Source: CAD feature listing. Evaluate the final solid. Frame: model axes, mm. Round coordinates to 2 decimals unless told otherwise and drop trailing zeros. Order: outer loops, then holes, each group sorted by start corner. A loop starts at its lowest first (then second) coordinate and runs counter-clockwise, first axis right, second up. Notation, with made-up numbers: (23, 52) - (58, 52) arc R20 cw to (58, 63) - close; hole circle Ø1 at (85, 87.5). An arc over 180 degrees is marked (long way). Put each result on its own line as item: value. Start each with the question number.
1) Line query: probe 1 along Z at (x, y) = (74.25, -88.5); probe 2 along X at (y, z) = (-58.5, 60); probe 3 along Y at (x, z) = (65.75, 38). Output: solid intervals per line, ascending. Write a range as [from, to].
2) Section A-A on y = -99. Output: boundary loops of the cut face in (x, z), then the cut area to 3 significant figures.
3) Section B-B on z = 41.75. Output: boundary loops of the cut face in (x, y).
4) Section D-D on y = -8. Output: boundary loops of the cut face in (x, z), then the cut area to 3 significant figures.
5) Contact query for flat-ended pins moving along their axis: P1, Ø1.5, axis at x = 69.5, z = 25.5, coming from the +Y side; P2, Ø2, axis at x = 63, y = 5, coming from the -Z side; P3, Ø1.3, axis at x = 65.5, y = -112.5, coming from the +Z side; P4, Ø9, axis at x = 65, z = 42, coming from the +Y side. Output: stop coordinate, or through.
6) Section C-C on z = 79.5. Output: boundary loops of the cut face in (x, y), then the cut area to 3 significant figures.
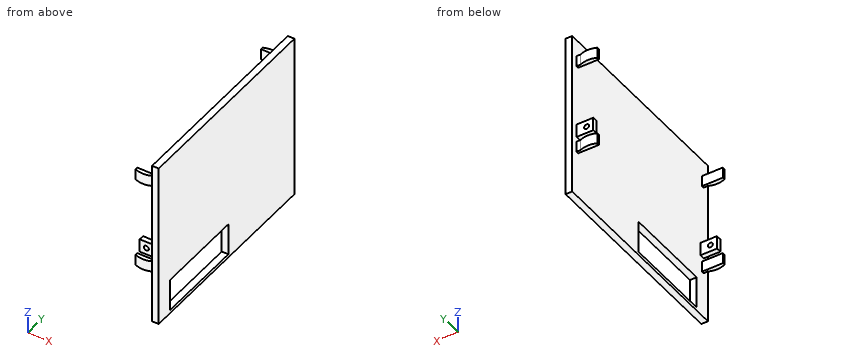
```python
from build123d import *

# Parameters (mm, degrees)
SKETCH2_W               = 4
SKETCH2_H               = 125
BOSS_EXTRUDE2_DEPTH     = 100
CUT_EXTRUDE1_REACH      = 132.347
SKETCH6_W               = 53.8
SKETCH6_H               = 19.347608653
SKETCH9_W               = 6.5
SKETCH9_H               = 1.5
BOSS_EXTRUDE4_DEPTH     = 12.5
BOSS_EXTRUDE5_DEPTH     = 6.5
LPATTERN2_COUNT         = 2
LPATTERN2_PITCH         = 55
MIRROR1_COPY_1_SKETCH_W = 6.5
MIRROR1_COPY_1_SKETCH_H = 1.5
MIRROR1_COPY_1_DEPTH    = 12.5
MIRROR1_COPY_2_DEPTH    = 6.5
SKETCH11_W              = 8
SKETCH11_H              = 3
BOSS_EXTRUDE6_DEPTH     = 10
SKETCH12_R              = 1.5
CUT_EXTRUDE2_DEPTH      = 3


with BuildPart() as part:
    # Sketch2 → Boss-Extrude2 (new body)
    with BuildSketch(Plane.XY):
        with Locations((72.870528802, -53.540266993)):
            Rectangle(SKETCH2_W, SKETCH2_H)
    extrude(amount=BOSS_EXTRUDE2_DEPTH)

    # Sketch6 → Cut-Extrude1 (cut, up to next)
    with BuildSketch(Plane(origin=(70.870528802, -52.340678406, -13.65152284), x_dir=(0, 1, 0), z_dir=(-1, 0, 0)), mode=Mode.PRIVATE) as cut_extrude1_sk1:
        with Locations((-26.429588587, -25.325327166)):
            Rectangle(SKETCH6_W, SKETCH6_H)
    cut_extrude1_tool1 = extrude(cut_extrude1_sk1.sketch, amount=-CUT_EXTRUDE1_REACH, mode=Mode.PRIVATE) & part.part
    add(cut_extrude1_tool1.solids().sort_by_distance((70.870529, -78.770267, 11.673804))[0], mode=Mode.SUBTRACT)

    # Sketch9 → Boss-Extrude4 (add)
    with BuildSketch(Plane.ZY.offset(-70.870528802)):
        with Locations((86.5, -111.290266993)):
            Rectangle(SKETCH9_W, SKETCH9_H)
    boss_extrude4 = extrude(amount=BOSS_EXTRUDE4_DEPTH)

    # Sketch10 → Boss-Extrude5 (add)
    with BuildSketch(Plane.XY.offset(89.75)):
        with BuildLine():
            Line((58.370528802, -112.040266993), (68.370528802, -112.040266993))
            ThreePointArc((68.370528802, -112.040266993), (63.370528802, -113.131554878), (58.370528802, -112.040266993))
        make_face()
    boss_extrude5 = extrude(amount=-BOSS_EXTRUDE5_DEPTH)

    # LPattern2: Boss-Extrude4, Boss-Extrude5 ×2
    with Locations(*[(0, 0, -i * LPATTERN2_PITCH) for i in range(1, LPATTERN2_COUNT)]):
        add(boss_extrude4)
        add(boss_extrude5)

    # Mirror1: Boss-Extrude4, Boss-Extrude5 across plane
    add(boss_extrude4.mirror(Plane.ZX.offset(-53.540266993)))
    add(boss_extrude5.mirror(Plane.ZX.offset(-53.540266993)))

    # Mirror1 copy 1 sketch → Mirror1 copy 1 (add)
    with BuildSketch(Plane(origin=(70.870528802, -107.080533985, -55), x_dir=(0, 0, 1), z_dir=(-1, 0, 0))):
        with Locations((86.5, 111.290266993)):
            Rectangle(MIRROR1_COPY_1_SKETCH_W, MIRROR1_COPY_1_SKETCH_H)
    extrude(amount=MIRROR1_COPY_1_DEPTH)

    # Mirror1 copy 2 sketch → Mirror1 copy 2 (add)
    with BuildSketch(Plane(origin=(0, -107.080533985, 34.75), x_dir=(1, 0, 0), z_dir=(0, 0, 1))):
        with BuildLine():
            Line((58.370528802, 112.040266993), (68.370528802, 112.040266993))
            ThreePointArc((68.370528802, 112.040266993), (63.370528802, 113.131554878), (58.370528802, 112.040266993))
        make_face()
    extrude(amount=-MIRROR1_COPY_2_DEPTH)

    # Sketch11 → Boss-Extrude6 (add)
    with BuildSketch(Plane.ZY.offset(-70.870528802)):
        with Locations((41.75, -110.540266993)):
            Rectangle(SKETCH11_W, SKETCH11_H)
    boss_extrude6 = extrude(amount=BOSS_EXTRUDE6_DEPTH)

    # Sketch12 → Cut-Extrude2 (cut)
    with BuildSketch(Plane(origin=(0, -112.040266993, 0), x_dir=(-1, 0, 0), z_dir=(0, -1, 0))):
        with Locations(Location((-64.870528802, -41.75, 0), (0, 0, 180))):
            Circle(SKETCH12_R)
    cut_extrude2 = extrude(amount=-CUT_EXTRUDE2_DEPTH, mode=Mode.SUBTRACT)

    # Mirror2: Boss-Extrude6, Cut-Extrude2 across plane
    add(boss_extrude6.mirror(Plane.ZX.offset(-53.540266993)))
    add(cut_extrude2.mirror(Plane.ZX.offset(-53.540266993)), mode=Mode.SUBTRACT)


solid = part.part
```
Answer sheet:
1. probe 1: [0, 2], [21.35, 100]
1. probe 2: [70.87, 74.87]
1. probe 3: [-112.04, -109.04], [1.96, 4.96]
2. outline: (70.87, 0) - (74.87, 0) - (74.87, 2) - (70.87, 2) - close; (70.87, 21.35) - (74.87, 21.35) - (74.87, 100) - (70.87, 100) - close
2. area: 323 mm^2
3. outline: (60.87, -112.04) - (63.37, -112.04) - (63.37, -109.04) - (60.87, -109.04) - close; (60.87, 1.96) - (63.37, 1.96) - (63.37, 4.96) - (60.87, 4.96) - close; (66.37, -112.04) - (70.87, -112.04) - (70.87, -116.04) - (74.87, -116.04) - (74.87, 8.96) - (70.87, 8.96) - (70.87, 4.96) - (66.37, 4.96) - (66.37, 1.96) - (70.87, 1.96) - (70.87, -109.04) - (66.37, -109.04) - close
4. outline: (70.87, 0) - (74.87, 0) - (74.87, 100) - (70.87, 100) - close
4. area: 400 mm^2
5. P1: through
5. P2: z = 28.25
5. P3: z = 89.75
5. P4: y = 4.96
6. outline: (70.87, -116.04) - (74.87, -116.04) - (74.87, 8.96) - (70.87, 8.96) - close
6. area: 500 mm^2
